Design review of the part built by this model. Coordinates are the model's own, in mm. A direction names the side the tool comes from. Coordinates: 2 decimals unless noted, no trailing zeros.
Q1. The part is to be moulded in two halves that separate along X. For faces 1 (the flat face through (14, -146.751, 3)), 2 (the flat face through (-118.646, -64, 3)), 3 (the flat face through (4, -196.751, 3)), say which applies: released by +X, released by -X, zero draft, split by the parting line, or undercut.
Q2. Take a section at A-A, the plane z = 3.25. State how many separate pieces and enclosed holes the cut face has, plus the area to 4 significant figures.
Q3. For L1, parallel to Y at x = -13, z = 5.25; L2, parallel to X at y = -134.5, z = 5.6; L3, parallel to X at y = -186, z = 5.55, list the stretches that pass through material, from the lowest coordinate up.
Q4. For faces 4 (the flat face through (14, -126.751, 3)), 5 (the flat face through (0, -60, 6)), list the 3-axis set-ups (+Z, -Z, +X, -X, +Y, -Y) from which the entire face can be reached by the end or side of a thin tool; tool diameter is ignored.
Autodesk Inventor part; units mm, degrees
ref_plane "YZ Plane" through (0, 0, 0) normal (1, 0, 0) x (0, 1, 0)
ref_plane "XZ Plane" through (0, 0, 0) normal (0, 1, 0) x (-1, 0, 0)
ref_plane "XY Plane" through (0, 0, 0) normal (0, 0, 1) x (1, 0, 0)
sketch "Sketch1" plane through (0, 0, 0) normal (0, 0, 1) x (1, 0, 0)
  line L0 (-118.6456, 73.2494) -> (122.9544, 73.2494)
  line L1 (122.9544, 73.2494) -> (122.9544, -196.7506)
  line L2 (122.9544, -196.7506) -> (-118.6456, -196.7506)
  line L3 (-118.6456, -196.7506) -> (-118.6456, 73.2494)
  circle A0 centre (-108.6456, 63.2494) radius 1.5
  circle A1 centre (112.9544, 63.2494) radius 1.5
  circle A2 centre (-108.6456, -186.7506) radius 1.5
  circle A3 centre (112.9544, -186.7506) radius 1.5
  point P0 (0, 0)
  dimension "d0" = 241.6
  dimension "d1" = 270
  dimension "d2" = 10
  dimension "d3" = 10
  dimension "d4" = 3
  dimension "d5" = 10
  dimension "d6" = 10
  dimension "d7" = 3
  dimension "d8" = 10
  dimension "d9" = 10
  dimension "d10" = 3
  dimension "d11" = 10
  dimension "d12" = 10
  dimension "d13" = 3
extrude "Extrusion1" add sketch "Sketch1" along normal blind 6
fillet "Fillet1" radius 4 4 edges at (-118.6456, 73.2494, 3) (122.9544, 73.2494, 3) (122.9544, -196.7506, 3) (-118.6456, -196.7506, 3)
sketch "Sketch2" plane through (0, 0, 0) normal (0, 0, -1) x (-1, 0, 0)
  line L0 (-22.9544, 3.2494) -> (-4.9544, 3.2494)
  line L1 (-4.9544, 3.2494) -> (-4.9544, -16.7506)
  line L2 (-4.9544, -16.7506) -> (-22.9544, -16.7506)
  line L3 (-22.9544, -16.7506) -> (-22.9544, 3.2494)
  line L4 (18.6456, -16.7506) -> (0.6456, -16.7506)
  line L5 (0.6456, -16.7506) -> (0.6456, 3.2494)
  line L6 (0.6456, 3.2494) -> (18.6456, 3.2494)
  line L7 (18.6456, 3.2494) -> (18.6456, -16.7506)
  line L8 (-22.9544, -146.7506) -> (-4.9544, -146.7506)
  line L9 (-4.9544, -146.7506) -> (-4.9544, -126.7506)
  line L10 (-4.9544, -126.7506) -> (-22.9544, -126.7506)
  line L11 (-22.9544, -126.7506) -> (-22.9544, -146.7506)
  line L12 (0.6456, -126.7506) -> (18.6456, -126.7506)
  line L13 (18.6456, -126.7506) -> (18.6456, -146.7506)
  line L14 (18.6456, -146.7506) -> (0.6456, -146.7506)
  line L15 (0.6456, -146.7506) -> (0.6456, -126.7506)
  line L16 (-122.9544, -192.7506) -> (-122.9544, 69.2494)
  line L17 (-118.9544, 73.2494) -> (114.6456, 73.2494)
  line L18 (118.6456, 69.2494) -> (118.6456, -192.7506)
  line L19 (114.6456, -196.7506) -> (-118.9544, -196.7506)
  point P0 (0, 0)
  dimension "d17" = 100
  dimension "d18" = 18
  dimension "d19" = 20
  dimension "d20" = 70
  dimension "d21" = 18
  dimension "d22" = 100
  dimension "d23" = 20
  dimension "d24" = 70
  dimension "d25" = 70
  dimension "d26" = 70
  dimension "d27" = 100
  dimension "d28" = 100
  dimension "d29" = 20
  dimension "d30" = 18
  dimension "d31" = 20
extrude "Extrusion3" cut sketch "Sketch2" against normal blind 6
properties part number "Etage 1"
Responses:
1. face 1: undercut
1. face 2: released by -X
1. face 3: zero draft
2. separate pieces: 1
2. enclosed holes: 8
2. area: 63,750 mm2
3. L1: y = -196.75 to -146.75, -126.75 to -16.75, 3.25 to 73.25
3. L2: x = -118.65 to -18.65, -0.65 to 4.95, 22.95 to 122.95
3. L3: x = -118.65 to -109.94, -107.35 to 111.66, 114.25 to 122.95
4. face 4: +Z, -Z
4. face 5: +Z, +X, -X, +Y, -Y
